Check sheet for the modelled part. Datum: model origin and axes. Units: mm. A direction names the side the tool comes from. Round coordinates to 2 decimals unless told otherwise and drop trailing zeros. Write each loop counter-clockwise with the first axis right and the second up, starting at its lowest first coordinate (ties: lowest second). Pieces come first, ordered by that corner, then holes. Notation, with made-up numbers: M 64.5,42.5 L 114.5,42.5 A19 cw 114.5,77.5 Z; hole C -39,38.5 d6. An arc over 180 degrees is marked long. Answer in a Markdown table with one row per item.
```python
from build123d import *

# Parameters (mm, degrees)
ESQUISSE1_R        = 15.7
ESQUISSE1_R_2      = 10.3
BOSS_EXTRU_1_DEPTH = 2
ESQUISSE2_R        = 20
ESQUISSE2_R_2      = 15.7
ESQUISSE2_R_3      = 10.3
BOSS_EXTRU_3_DEPTH = 2
ECHELLE1_SCALE     = 2
ECHELLE2_SCALE     = 0.25


with BuildPart() as part:
    # Esquisse1 → Boss.-Extru.1 (new body)
    with BuildSketch(Plane.XY):
        Circle(ESQUISSE1_R)
        Circle(ESQUISSE1_R_2, mode=Mode.SUBTRACT)
    extrude(amount=BOSS_EXTRU_1_DEPTH)

    # Esquisse2 → Boss.-Extru.3 (add)
    # profile 1 of 2: a face of its own
    with BuildSketch(Plane.XY.offset(2)):
        Circle(ESQUISSE2_R)
        Circle(ESQUISSE2_R_2, mode=Mode.SUBTRACT)
    # profile 2 of 2: a face of its own
    with BuildSketch(Plane.XY.offset(2)):
        Circle(ESQUISSE2_R_2)
        Circle(ESQUISSE2_R_3, mode=Mode.SUBTRACT)
    extrude(amount=BOSS_EXTRU_3_DEPTH)


with BuildPart() as part_1:
    # Echelle1: scaled about (0, 0, 2.353457208)
    add(part.part.scale(ECHELLE1_SCALE).moved(Location((0, 0, -2.353457208))))


with BuildPart() as part_2:
    # Echelle2: scaled about (0, 0, 2.353457208)
    add(part_1.part.scale(ECHELLE2_SCALE).moved(Location((0, 0, 1.765092906))))


solid = part_2.part
```
1. Scan lines: L1, parallel to Y at x = 0, z = 2.1; L2, parallel to Y at x = 2.5, z = 2.25; L3, parallel to X at y = 4.75, z = 1.95. Record each from-to range of solid material in increasing order.
Found:
| item | result |
|---|---|
| L1 | y = -7.85 to -5.15, 5.15 to 7.85 |
| L2 | y = -9.68 to -4.5, 4.5 to 9.68 |
| L3 | x = -6.25 to -1.99, 1.99 to 6.25 |
2. Section check D-D, the plane z = 1.5. Record the cut outline in (x, y).
Found:
| item | result |
|---|---|
| outline | C 0,0 d15.7; hole C 0,0 d10.3 |
3. Draft check along X on faces 1 (the face through (4.91, 1.55, 2.16)), 2 (the face through (-5.786, 5.305, 1.67)), 3 (the face through (5, -2, 1.177)). Enter one of: +X half, -X half, draft (parallel to the pull), parting line (faces both ways), or undercut.
Found:
| item | result |
|---|---|
| face 1 | undercut |
| face 2 | parting line |
| face 3 | draft |
4. Go/stop test with flat-tipped pins: pin 1 (1 mm diameter, centred on y = 2, z = 2, fed in from +X); pin 2 (1 mm diameter, centred on x = -3, z = 2, fed in from -Y). Record where each tip stops, or that it passes through.
Found:
| item | result |
|---|---|
| pin 1 | stops at x = 9.88 |
| pin 2 | stops at y = -9.67 |
5. Access from +Z, -Z, +X, -X, +Y, -Y to the whole of each face (thin tool, end or side, straight path). Record for faces 4 (the face through (4, -7, 2.177)), 5 (the face through (-2, 5, 3.177)).
Found:
| item | result |
|---|---|
| face 4 | -Z |
| face 5 | +Z, +X, -X, +Y, -Y |
6. Section check A-A, the plane y = 0. Record the cut outline in (x, z), and give its area (3 significant figures).
Found:
| item | result |
|---|---|
| outline | M -10,2.18 L -7.85,2.18 L -7.85,1.18 L -5.15,1.18 L -5.15,3.18 L -10,3.18 Z; M 5.15,1.18 L 7.85,1.18 L 7.85,2.18 L 10,2.18 L 10,3.18 L 5.15,3.18 Z |
| area | 15.1 mm2 |
7. Section check C-C, the plane y = -6.75. Record the cut outline in (x, z), and give its area (3 significant figures).
Found:
| item | result |
|---|---|
| outline | M -7.38,2.18 L -4.01,2.18 L -4.01,1.18 L 4.01,1.18 L 4.01,2.18 L 7.38,2.18 L 7.38,3.18 L -7.38,3.18 Z |
| area | 22.8 mm2 |
